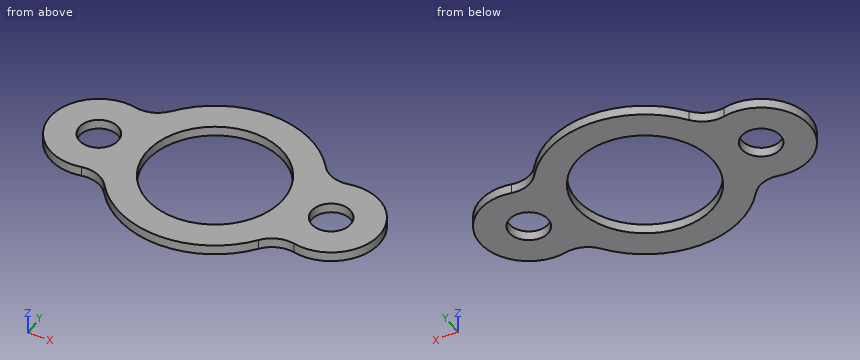
```python
from build123d import *

# Parameters (mm, degrees)
F0_R     = 12.7
F0_R_2   = 44.45
F1_DEPTH = 6.35


with BuildPart() as f1:
    # F0 (on Top) → F1 (new body)
    with BuildSketch(Plane.XY):
        with BuildLine():
            ThreePointArc((-50.825601, 38.253471), (-59.266449, 31.925086), (-69.783439, 31.094859))
            ThreePointArc((-69.783439, 31.094859), (-107.949998, -0.010447), (-69.762979, -31.09063))
            ThreePointArc((-69.762979, -31.09063), (-69.761122, -31.090245), (-69.759266, -31.089861))
            ThreePointArc((-69.759266, -31.089861), (-59.198353, -31.914391), (-50.716273, -38.260023))
            Line((-50.716273, -38.260023), (-50.692897, -38.242388))
            ThreePointArc((-50.692897, -38.242388), (-0.01246, -63.499999), (50.677885, -38.262279))
            ThreePointArc((50.677885, -38.262279), (59.174451, -31.910614), (69.750781, -31.088102))
            ThreePointArc((69.750781, -31.088102), (107.95, 0), (69.750781, 31.088102))
            ThreePointArc((69.750781, 31.088102), (59.174451, 31.910614), (50.677885, 38.262279))
            ThreePointArc((50.677885, 38.262279), (-0.047933, 63.499982), (-50.735592, 38.185726))
            Line((-50.735592, 38.185726), (-50.825601, 38.253471))
        make_face()
        with Locations((-76.2, 0)):
            Circle(F0_R, mode=Mode.SUBTRACT)
        Circle(F0_R_2, mode=Mode.SUBTRACT)
        with Locations((76.2, 0)):
            Circle(F0_R, mode=Mode.SUBTRACT)
    extrude(amount=F1_DEPTH)


solid = f1.part
```
Work out the finished part from the listing and answer in its coordinate system (mm). Coordinates: 2 decimals unless noted, no trailing zeros. Write each loop counter-clockwise with the first axis right and the second up, starting at its lowest first coordinate (ties: lowest second). Pieces come first, ordered by that corner, then holes.
Q1. A cutting plane is placed at C-C, the plane z = 3.5. State how many separate pieces and enclosed holes the cut face has, then the cut area to 3 significant figures.
Q2. A cutting plane is placed at A-A, the plane x = 0. Give the vertices of the cut face in (y, z), then the cut area to 3 significant figures.
Q3. A cutting plane is placed at D-D, the plane x = 61. Give the vertices of the cut face in (y, z), then the cut area to 3 significant figures.
Q4. Find the intervals of material crossed by line 1 (Y direction, x = 76.2, z = 4.75); line 2 (Y direction, x = 0, z = 3.75); line 3 (X direction, y = -10, z = 5), in increasing order.
Q5. Each of these flat-tipped pins is pushed along its axis until it touches: pin 1 Ø20.5 at (x, y) = (-76.2, 0) entering from -Z; pin 2 Ø2 at (x, z) = (77.5, 2) entering from -Y; pin 3 Ø1 at (x, z) = (-61.5, 4) entering from -Y. Where does it stop, or does it pass through?
Q6. A cutting plane is placed at B-B, the plane y = 18.5. Give the vertices of the cut face in (x, z), then the cut area to 3 significant figures.
Findings below:
1. separate pieces: 1
1. enclosed holes: 3
1. area: 10,600 mm2
2. outline: (-63.5, 0) - (-44.45, 0) - (-44.45, 6.35) - (-63.5, 6.35) - close; (44.45, 0) - (63.5, 0) - (63.5, 6.35) - (44.45, 6.35) - close
2. area: 242 mm2
3. outline: (-31.33, 0) - (31.33, 0) - (31.33, 6.35) - (-31.33, 6.35) - close
3. area: 398 mm2
4. line 1: y = -31.75 to -12.7, 12.7 to 31.75
4. line 2: y = -63.5 to -44.45, 44.45 to 63.5
4. line 3: x = -106.33 to -84.03, -68.37 to -43.31, 43.31 to 68.37, 84.03 to 106.33
5. pin 1: passes through
5. pin 2: stops at y = -31.75
5. pin 3: stops at y = -31.34
6. outline: (-102, 0) - (-40.42, 0) - (-40.42, 6.35) - (-102, 6.35) - close; (40.42, 0) - (102, 0) - (102, 6.35) - (40.42, 6.35) - close
6. area: 782 mm2
